```python
from build123d import *

# Parameters (mm, degrees)
SKETCH_R      = 29
SKETCH_R_2    = 1.6
PAD_DEPTH     = 4
SKETCH001_R   = 15
PAD001_DEPTH  = 21
SKETCH002_R   = 13
POCKET_DEPTH  = 40
SKETCH003_R   = 13
SKETCH003_R_2 = 1.6
PAD002_DEPTH  = 4
FILLET_R      = 2


with BuildPart() as part:
    # Sketch → Pad (new body)
    with BuildSketch(Plane.XY):
        Circle(SKETCH_R)
        with Locations((0, 24)):
            Circle(SKETCH_R_2, mode=Mode.SUBTRACT)
        with Locations((20.78461, -12)):
            Circle(SKETCH_R_2, mode=Mode.SUBTRACT)
        with Locations((-20.78461, -12)):
            Circle(SKETCH_R_2, mode=Mode.SUBTRACT)
    extrude(amount=PAD_DEPTH)

    # Sketch001 (on Face6 of Pad) → Pad001 (join)
    with BuildSketch(Plane.XY.offset(4)):
        Circle(SKETCH001_R)
    extrude(amount=PAD001_DEPTH)

    # Sketch002 (on Face8 of Pad001) → Pocket (cut)
    with BuildSketch(Plane.XY.offset(25)):
        Circle(SKETCH002_R)
    extrude(amount=-POCKET_DEPTH, mode=Mode.SUBTRACT)

    # Sketch003 (on Face9 of Pocket) → Pad002 (join)
    with BuildSketch(Plane.XY.offset(25)):
        with BuildLine():
            ThreePointArc((-14.672214, 3.118675), (0, -15), (14.672214, 3.118675))
            Line((14.672214, 3.118675), (22.497395, 4.781969))
            ThreePointArc((22.497395, 4.781969), (0, 23), (-22.497395, 4.781969))
            Line((-14.672214, 3.118675), (-22.497395, 4.781969))
        make_face()
        Circle(SKETCH003_R, mode=Mode.SUBTRACT)
        with Locations((-17.5, 8)):
            Circle(SKETCH003_R_2, mode=Mode.SUBTRACT)
        with Locations((17.5, 8)):
            Circle(SKETCH003_R_2, mode=Mode.SUBTRACT)
    extrude(amount=PAD002_DEPTH)

    # Fillet
    fillet_edges = [part.edges().sort_by_distance(p)[0] for p in [
        (22.497395, 4.781969, 27),
        (-22.497395, 4.781969, 27),
    ]]
    fillet(fillet_edges, radius=FILLET_R)


solid = part.part
```
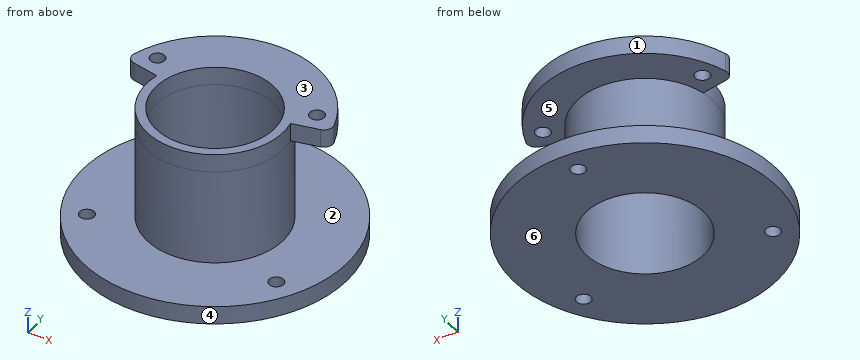
The listing builds one solid part. Answer for the finished solid, in the listing's coordinates (mm). Face numbers are marked on the shaded views. A direction names the side the tool comes from. Coordinates: 2 decimals unless noted, no trailing zeros. Loops run counter-clockwise (first coordinate to the right, second up) from the corner with the lowest first, then second, coordinate; pieces in that order, holes last. Notation, with made-up numbers: (-3.75, -19) - (22.25, -19) arc R14 cw to (22.25, 4) - close; hole circle Ø4 at (-12, -0.5). An arc over 180 degrees is marked (long way). Write item = value, one per line.
1) Each of these flat-tipped pins is pushed along its axis until it touches: P1, Ø1.5, axis at y = 6, z = 23.5, coming from the +X side; P2, Ø5, axis at x = 6.5, y = -17, coming from the +Z side; P3, Ø2.5, axis at x = 0, y = 24, coming from the -Z side; P4, Ø5, axis at x = -20.78, y = -12, coming from the -Z side. Where does it stop, or does it pass through?
Responses:
P1 = 14.05
P2 = 4
P3 = 25
P4 = 0
2) Find the intervals of material crossed by line 1 along Y through (x, z) = (0, 1.95); line 2 along Z through (x, y) = (21, 14); line 3 along Y through (x, z) = (11.5, 19.75), in increasing order.
Responses:
line_1 = -29 to -13, 13 to 22.4, 25.6 to 29
line_2 = 0 to 4
line_3 = -9.63 to -6.06, 6.06 to 9.63
3) Section A-A (y = 0) is taken. Determine the outline of the cut face in (x, z).
Responses:
outline = (-29, 0) - (-13, 0) - (-13, 29) - (-15, 29) - (-15, 4) - (-29, 4) - close; (13, 0) - (29, 0) - (29, 4) - (15, 4) - (15, 29) - (13, 29) - close
4) Which of the six approach directions +Z, -Z, +X, -X, +Y, -Y give full straight-line access (tool end or side, diameter ignored) to the marked faces 1 and 2?
Responses:
face_1 = +Z, +Y
face_2 = none
5) Section C-C (z = 6) is taken. Determine the outline of the cut face in (x, y).
Responses:
outline = circle Ø30 at (0, 0); hole circle Ø26 at (0, 0)
6) Section D-D (x = 9) is taken. Determine the outline of the cut face in (y, z), plus the area to 3 significant figures.
Responses:
outline = (-27.57, 0) - (-9.38, 0) - (-9.38, 29) - (-12, 29) - (-12, 4) - (-27.57, 4) - close; (9.38, 0) - (27.57, 0) - (27.57, 4) - (12, 4) - (12, 25) - (21.17, 25) - (21.17, 29) - (9.38, 29) - close
area = 313 mm^2
7) Determine the mould class of the marked faces 3, 4, 5 and 6 for opening direction Z: pulls with the +Z half, pulls with the -Z half, needs draft (parallel to the pull), parting line crosses it, or undercut.
Responses:
face_3 = pulls with the +Z half
face_4 = needs draft
face_5 = undercut
face_6 = pulls with the -Z half
8) Section B-B (x = 0) is taken. Determine the outline of the cut face in (y, z), plus the area to 3 significant figures.
Responses:
outline = (-29, 0) - (-13, 0) - (-13, 29) - (-15, 29) - (-15, 4) - (-29, 4) - close; (13, 0) - (22.4, 0) - (22.4, 4) - (15, 4) - (15, 25) - (23, 25) - (23, 29) - (13, 29) - close; (25.6, 0) - (29, 0) - (29, 4) - (25.6, 4) - close
area = 247 mm^2
